The listing builds one solid part. Answer for the finished solid, in the listing's coordinates (mm). Face numbers are marked on the shaded views. A direction names the side the tool comes from. Give positions to 0.01 mm unless a question says otherwise; leave off trailing zeros. Write each loop counter-clockwise with the first axis right and the second up, starting at its lowest first coordinate (ties: lowest second). Pieces come first, ordered by that corner, then holes.
```python
from build123d import *

# Parameters (mm, degrees)
F1_DEPTH  = 20
F2_R      = 6
F2_R_2    = 2.75
F3_DEPTH  = 20.001
F4_R      = 5.4
F5_DEPTH  = 1.5
F6_R      = 3.3
F7_DEPTH  = 31.001
F8_R      = 12.0269
F9_DEPTH  = 6
F10_R     = 11.6713
F11_DEPTH = 6
F12_SIZE  = 2.54
F13_SIZE  = 0.5


with BuildPart() as f1:
    # F0 (on Front) → F1 (new body)
    with BuildSketch(Plane.XZ):
        Polygon((-30, -16.25), (30, -16.25), (30, 16.25), (17, 16.25), (17, 23.75), (-17, 23.75), (-17, 16.25), (-30, 16.25), align=None)
    extrude(amount=F1_DEPTH)

    # F2 (on face) → F3 (cut, through all)
    with BuildSketch(Plane.XZ.offset(20)):
        with Locations((0, 8.75)):
            Circle(F2_R)
        with Locations((-23, 8.75)):
            Circle(F2_R_2)
        with Locations((-23, -9.25)):
            Circle(F2_R_2)
        with Locations((23, 8.75)):
            Circle(F2_R_2)
        with Locations((23, -9.25)):
            Circle(F2_R_2)
    extrude(amount=-F3_DEPTH, mode=Mode.SUBTRACT)

    # F4 (on face) → F5 (cut)
    with BuildSketch(Plane.XY.offset(16.25)):
        with Locations((-23, -10)):
            Circle(F4_R)
        with Locations((23, -10)):
            Circle(F4_R)
    extrude(amount=-F5_DEPTH, mode=Mode.SUBTRACT)

    # F6 (on face) → F7 (cut, through all)
    with BuildSketch(Plane.XY.offset(14.75)):
        with Locations((-23, -10)):
            Circle(F6_R)
        with Locations((23, -10)):
            Circle(F6_R)
    extrude(amount=-F7_DEPTH, mode=Mode.SUBTRACT)

    # F8 (on face) → F9 (cut)
    with BuildSketch(Plane.XZ.offset(20)):
        with Locations((0, 8.75)):
            Circle(F8_R)
    extrude(amount=-F9_DEPTH, mode=Mode.SUBTRACT)

    # F10 (on face) → F11 (cut)
    with BuildSketch(Plane(origin=(0, 0, 0), x_dir=(-1, 0, 0), z_dir=(0, 1, 0))):
        with Locations((0, 8.75)):
            Circle(F10_R)
    extrude(amount=-F11_DEPTH, mode=Mode.SUBTRACT)

    # F12
    f12_edges = [f1.edges().sort_by_distance(p)[0] for p in [
        (17, -10, 23.75),
        (-17, -10, 23.75),
    ]]
    chamfer(f12_edges, length=F12_SIZE)

    # F13
    f13_edges = [f1.edges().sort_by_distance(p)[0] for p in [
        (23.5, 0, 16.25),
        (17, 0, 18.73),
        (15.73, 0, 22.48),
        (0, 0, 23.75),
        (-15.73, 0, 22.48),
        (-17, 0, 18.73),
        (-23.5, 0, 16.25),
        (-30, 0, 0),
        (0, 0, -16.25),
        (30, 0, 0),
        (30, -10, 16.25),
        (30, -20, 0),
        (30, -10, -16.25),
        (23.5, -20, 16.25),
        (17, -20, 18.73),
        (15.73, -20, 22.48),
        (0, -20, 23.75),
        (-15.73, -20, 22.48),
        (-17, -20, 18.73),
        (-23.5, -20, 16.25),
        (-30, -20, 0),
        (-30, -10, -16.25),
        (0, -20, -16.25),
    ]]
    chamfer(f13_edges, length=F13_SIZE)


solid = f1.part
```
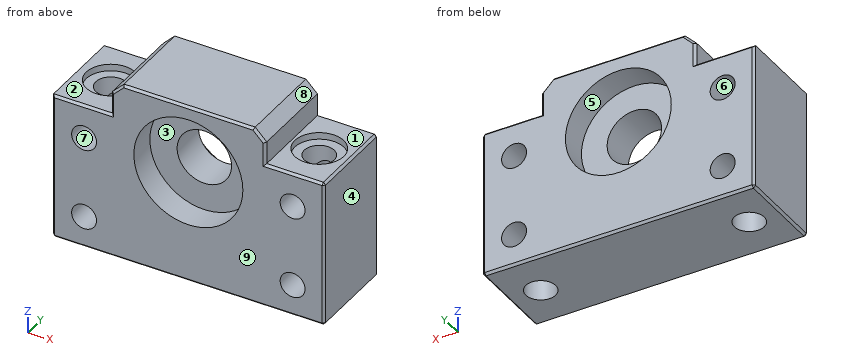
Item 1: Each of these flat-tipped pins is pushed along its axis until it touches: P1, Ø10.5, axis at x = -26, y = -12.5, coming from the +Z side; P2, Ø2, axis at x = 0.5, z = 17.5, coming from the -Y side; P3, Ø6.5, axis at x = 23, z = -9.25, coming from the -Y side; P4, Ø4, axis at y = -6, z = 18, coming from the +X side. Where does it stop, or does it pass through?
Conclusion:
P1: stops at z = 16.25
P2: stops at y = -14
P3: stops at y = -20
P4: stops at x = 29.75
Item 2: Which of the six approach directions +Z, -Z, +X, -X, +Y, -Y give full straight-line access (tool end or side, diameter ignored) to the marked faces 1, 2, 3, 4 and 5?
Conclusion:
face 1: +Z, +X, +Y, -Y
face 2: +Z, -X, +Y, -Y
face 3: -Y
face 4: +Z, -Z, +X, +Y, -Y
face 5: +Y
Item 3: A cutting plane is placed at B-B, the plane x = 0. Give the vertices of the cut face in (y, z).
Conclusion:
outline: (-20, -15.75) - (-19.5, -16.25) - (-0.5, -16.25) - (0, -15.75) - (0, -2.92) - (-6, -2.92) - (-6, 2.75) - (-14, 2.75) - (-14, -3.28) - (-20, -3.28) - close; (-20, 20.78) - (-14, 20.78) - (-14, 14.75) - (-6, 14.75) - (-6, 20.42) - (0, 20.42) - (0, 23.25) - (-0.5, 23.75) - (-19.5, 23.75) - (-20, 23.25) - close
Item 4: Determine the mould class of the marked faces 6, 7, 8 and 9 for opening direction Z: pulls with the +Z half, pulls with the -Z half, needs draft (parallel to the pull), parting line crosses it, or undercut.
Conclusion:
face 6: undercut
face 7: undercut
face 8: pulls with the +Z half
face 9: needs draft
Item 5: A cutting plane is placed at A-A, the plane z = -9.25. Give the vertices of the cut face in (x, y).
Conclusion:
outline: (-30, -19.5) - (-29.5, -20) - (-25.75, -20) - (-25.75, -11.82) arc R3.3 cw to (-25.75, -8.18) - (-25.75, 0) - (-29.5, 0) - (-30, -0.5) - close; (-20.25, -20) - (20.25, -20) - (20.25, -11.82) arc R3.3 cw to (20.25, -8.18) - (20.25, 0) - (-20.25, 0) - (-20.25, -8.18) arc R3.3 cw to (-20.25, -11.82) - close; (25.75, -20) - (29.5, -20) - (30, -19.5) - (30, -0.5) - (29.5, 0) - (25.75, 0) - (25.75, -8.18) arc R3.3 cw to (25.75, -11.82) - close
Item 6: A cutting plane is placed at C-C, the plane y = -10. Count the separate pieces of the cut face and the enclosed holes in it, plus the area to 3 significant figures.
Conclusion:
separate pieces: 3
enclosed holes: 1
area: 1,640 mm2
Item 7: Consider probe 1 along X at (y, z) = (-2, 9); probe 2 along Z at (x, y) = (-23, -6); probe 3 along X at (y, z) = (-17.5, 8.5). Determine where each line is inside the solid, lowest interval first.
Conclusion:
probe 1: x = -30 to -25.74, -20.26 to -11.67, 11.67 to 20.26, 25.74 to 30
probe 2: z = -16.25 to -12, -6.5 to 6, 11.5 to 14.75
probe 3: x = -30 to -25.74, -20.26 to -12.02, 12.02 to 20.26, 25.74 to 30
